```python
from build123d import *

# Parameters (mm, degrees)
BOSS_EXTRUDE1_DEPTH                        = 10
BOSS_EXTRUDE1_2_DEPTH                      = 10
SKETCH2_W                                  = 149
SKETCH2_H                                  = 57
BOSS_EXTRUDE2_DEPTH                        = 3
SKETCH3_W                                  = 125
SKETCH3_H                                  = 31
CUT_EXTRUDE1_DEPTH                         = 20
SKETCH4_W                                  = 20
SKETCH4_H                                  = 20
BOSS_EXTRUDE3_DEPTH                        = 3
SKETCH5_R                                  = 2
CUT_EXTRUDE2_DEPTH                         = 20
SKETCH6_R                                  = 4.5
CUT_EXTRUDE3_DEPTH                         = 2
MIRROR5_AT_THE_SECOND_PLANE_COPY_1_SKETC_W = 20
MIRROR5_AT_THE_SECOND_PLANE_COPY_1_SKETC_H = 20
MIRROR5_AT_THE_SECOND_PLANE_COPY_1_DEPTH   = 3
MIRROR5_AT_THE_SECOND_PLANE_COPY_2_SKETC_R = 2
MIRROR5_AT_THE_SECOND_PLANE_COPY_2_DEPTH   = 20
MIRROR5_AT_THE_SECOND_PLANE_COPY_3_SKETC_R = 4.5
MIRROR5_AT_THE_SECOND_PLANE_COPY_3_DEPTH   = 2
CHAMFER1_SIZE                              = 5


with BuildPart() as part:
    # Sketch1 → Boss-Extrude1 (new body)
    with BuildSketch(Plane(origin=(0, 0, 0), x_dir=(1, 0, 0), z_dir=(0, 1, 0))):
        Polygon((74.5, 28.5), (-74.5, 28.5), (-74.5, 23.5), (-69.5, 23.5), (69.5, 23.5), (74.5, 23.5), align=None)
    extrude(amount=BOSS_EXTRUDE1_DEPTH)



with BuildPart() as body_2:
    # Sketch1 → Boss-Extrude1 2 (new body)
    with BuildSketch(Plane(origin=(0, 0, 0), x_dir=(1, 0, 0), z_dir=(0, 1, 0))):
        Polygon((-69.5, -23.5), (-74.5, -23.5), (-74.5, -28.5), (74.5, -28.5), (74.5, -23.5), (69.5, -23.5), align=None)
    extrude(amount=BOSS_EXTRUDE1_2_DEPTH)


with BuildPart() as part_1:
    add(part.part)

    add(body_2.part)  # Boss-Extrude2 merges body 2
    # Sketch2 → Boss-Extrude2 (add)
    with BuildSketch(Plane.XZ):
        Rectangle(SKETCH2_W, SKETCH2_H)
    extrude(amount=BOSS_EXTRUDE2_DEPTH)

    # Sketch3 → Cut-Extrude1 (cut)
    with BuildSketch(Plane(origin=(0, 0, 0), x_dir=(1, 0, 0), z_dir=(0, 1, 0))):
        Rectangle(SKETCH3_W, SKETCH3_H)
    extrude(amount=-CUT_EXTRUDE1_DEPTH, mode=Mode.SUBTRACT)

    # Sketch4 → Boss-Extrude3 (add, symmetric)
    with BuildSketch(Plane(origin=(0, 0, 0), x_dir=(1, 0, 0), z_dir=(0, 1, 0))):
        with Locations((-64.5, 38.5)):
            Rectangle(SKETCH4_W, SKETCH4_H)
    boss_extrude3 = extrude(amount=BOSS_EXTRUDE3_DEPTH, both=True)

    # Sketch5 → Cut-Extrude2 (cut)
    with BuildSketch(Plane(origin=(0, 3, 0), x_dir=(1, 0, 0), z_dir=(0, 1, 0))):
        with Locations((-65, 38.5)):
            Circle(SKETCH5_R)
    cut_extrude2 = extrude(amount=-CUT_EXTRUDE2_DEPTH, mode=Mode.SUBTRACT)

    # Sketch6 → Cut-Extrude3 (cut)
    with BuildSketch(Plane(origin=(0, 3, 0), x_dir=(1, 0, 0), z_dir=(0, 1, 0))):
        with Locations((-65, 38.5)):
            Circle(SKETCH6_R)
    cut_extrude3 = extrude(amount=-CUT_EXTRUDE3_DEPTH, mode=Mode.SUBTRACT)

    # Mirror5: Boss-Extrude3, Cut-Extrude2, Cut-Extrude3 across plane
    add(boss_extrude3.mirror(Plane.XY))
    add(cut_extrude2.mirror(Plane.XY), mode=Mode.SUBTRACT)
    add(cut_extrude3.mirror(Plane.XY), mode=Mode.SUBTRACT)

    # Mirror5 at the second plane: Boss-Extrude3, Cut-Extrude3, Cut-Extrude2 across plane
    add(boss_extrude3.mirror(Plane(origin=(0, 0, 0), x_dir=(0, 0, 1), z_dir=(1, 0, 0))))
    add(cut_extrude3.mirror(Plane(origin=(0, 0, 0), x_dir=(0, 0, 1), z_dir=(1, 0, 0))), mode=Mode.SUBTRACT)
    add(cut_extrude2.mirror(Plane(origin=(0, 0, 0), x_dir=(0, 0, 1), z_dir=(1, 0, 0))), mode=Mode.SUBTRACT)

    # Mirror5 at the second plane copy 1 sketc → Mirror5 at the second plane copy 1 (add, symmetric)
    with BuildSketch(Plane(origin=(0, 0, 0), x_dir=(-1, 0, 0), z_dir=(0, 1, 0))):
        with Locations((-64.5, 38.5)):
            Rectangle(MIRROR5_AT_THE_SECOND_PLANE_COPY_1_SKETC_W, MIRROR5_AT_THE_SECOND_PLANE_COPY_1_SKETC_H)
    extrude(amount=MIRROR5_AT_THE_SECOND_PLANE_COPY_1_DEPTH, both=True)

    # Mirror5 at the second plane copy 2 sketc → Mirror5 at the second plane copy 2 (cut)
    with BuildSketch(Plane(origin=(0, 3, 0), x_dir=(-1, 0, 0), z_dir=(0, 1, 0))):
        with Locations((-65, 38.5)):
            Circle(MIRROR5_AT_THE_SECOND_PLANE_COPY_2_SKETC_R)
    extrude(amount=-MIRROR5_AT_THE_SECOND_PLANE_COPY_2_DEPTH, mode=Mode.SUBTRACT)

    # Mirror5 at the second plane copy 3 sketc → Mirror5 at the second plane copy 3 (cut)
    with BuildSketch(Plane(origin=(0, 3, 0), x_dir=(-1, 0, 0), z_dir=(0, 1, 0))):
        with Locations((-65, 38.5)):
            Circle(MIRROR5_AT_THE_SECOND_PLANE_COPY_3_SKETC_R)
    extrude(amount=-MIRROR5_AT_THE_SECOND_PLANE_COPY_3_DEPTH, mode=Mode.SUBTRACT)

    # Chamfer1
    chamfer1_edges = [part_1.edges().sort_by_distance(p)[0] for p in [
        (74.5, 0, 48.5),
        (54.5, 0, 28.5),
        (54.5, 0, 48.5),
        (64.5, 3, 28.5),
        (-74.5, 0, -48.5),
        (-54.5, 0, -28.5),
        (-54.5, 0, -48.5),
        (-64.5, 3, -28.5),
        (74.5, 0, -48.5),
        (54.5, 0, -48.5),
        (54.5, 0, -28.5),
        (64.5, 3, -28.5),
        (-74.5, 0, 48.5),
        (-54.5, 0, 48.5),
        (-54.5, 0, 28.5),
        (-64.5, 3, 28.5),
    ]]
    chamfer(chamfer1_edges, length=CHAMFER1_SIZE)


solid = part_1.part
```
Here's how the part is built. I have some questions about the finished solid (model axes, mm). A direction names the side the tool comes from. Round coordinates to 2 decimals unless told otherwise and drop trailing zeros. Write each loop counter-clockwise with the first axis right and the second up, starting at its lowest first coordinate (ties: lowest second). Pieces come first, ordered by that corner, then holes.
Q1. Will these pins go through, and if not, where does the flat tip stop? P1, Ø7, axis at x = 67, z = -40.5, coming from the +Y side; P2, Ø6, axis at x = 5.5, y = 5, coming from the +Z side; P3, Ø5, axis at x = -65, z = 38.5, coming from the +Y side.
Q2. If we section it at C-C on z = 38.5: Write out the boundary of the cut face in (x, y).
Q3. If we section it at A-A on z = -11: Write out the boundary of the cut face in (x, y).
Q4. If we section it at B-B on x = 22: Write out the boundary of the cut face in (y, z).
Q5. Please list where these lines run through material, in increasing order: probe 1 along Z at (x, y) = (-65, -1.95); probe 2 along X at (y, z) = (1.45, -38.5); probe 3 along Z at (x, y) = (-58.5, 9.5).
Q6. Which directions (+Z, -Z, +X, -X, +Y, -Y) give clear straight access to the entire face, cutting with the end or side of a thin tool? Please do faces 4 (the flat face through (-62.5, -1, 0)), 5 (the flat face through (62, 3, -43)), 6 (the flat face through (-62, 3, 43)), 7 (the flat face through (52, 1, 31)), 8 (the cylindrical face through (62.92, 2.01, -34.51)).
Q7. If we section it at D-D on y = 5.5: Write out the boundary of the cut face in (x, z), plus the area to 3 significant figures.
Q8. If we mould it in two halves opening along Z, with no side actions, what happens to faces 1 (the flat face through (-62.2, 5.5, -31)), 2 (the cylindrical face through (-62.92, 2.01, 34.51)), 3 (the flat face through (-62, 3, -43))? For each: +Z half, -Z half, draft (parallel to the pull), parting line (faces both ways), or undercut.
Answer below:
1. P1: stops at y = 3
1. P2: stops at z = 28.5
1. P3: stops at y = 1
2. outline: (-74.5, -3) - (-67, -3) - (-67, 1) - (-69.5, 1) - (-69.5, 3) - (-74.5, 3) - close; (-63, -3) - (-54.5, -3) - (-54.5, 3) - (-60.5, 3) - (-60.5, 1) - (-63, 1) - close; (54.5, -3) - (63, -3) - (63, 1) - (60.5, 1) - (60.5, 3) - (54.5, 3) - close; (67, -3) - (74.5, -3) - (74.5, 3) - (69.5, 3) - (69.5, 1) - (67, 1) - close
3. outline: (-74.5, -3) - (-62.5, -3) - (-62.5, 0) - (-74.5, 0) - close; (62.5, -3) - (74.5, -3) - (74.5, 0) - (62.5, 0) - close
4. outline: (-3, -28.5) - (10, -28.5) - (10, -23.5) - (0, -23.5) - (0, -15.5) - (-3, -15.5) - close; (-3, 15.5) - (0, 15.5) - (0, 23.5) - (10, 23.5) - (10, 28.5) - (-3, 28.5) - close
5. probe 1: z = -48.5 to -40.5, -36.5 to 36.5, 40.5 to 48.5
5. probe 2: x = -74.5 to -69.5, -60.5 to -54.5, 54.5 to 60.5, 69.5 to 74.5
5. probe 3: z = -28.5 to -23.5, 23.5 to 28.5
6. face 4: +Y, -Y
6. face 5: -Z, +X, -X, +Y
6. face 6: +Z, +X, -X, +Y
6. face 7: +Z, +Y, -Y
6. face 8: +Y
7. outline: (-74.5, -31) - (-52, -31) - (-49.5, -28.5) - (49.5, -28.5) - (52, -31) - (74.5, -31) - (74.5, -23.5) - (-74.5, -23.5) - close; (-74.5, 23.5) - (74.5, 23.5) - (74.5, 31) - (52, 31) - (49.5, 28.5) - (-49.5, 28.5) - (-52, 31) - (-74.5, 31) - close
7. area: 1,730 mm2
8. face 1: -Z half
8. face 2: undercut
8. face 3: draft
